```python
from build123d import *

# Parameters (mm, degrees)
SKETCH_W               = 7.5
SKETCH_H               = 7.5
PAD_DEPTH              = 10
POCKET_DEPTH           = 7.501
LINEARPATTERN_COUNT    = 2
LINEARPATTERN_PITCH    = 2.4
LINEARPATTERN001_COUNT = 2
LINEARPATTERN001_PITCH = 2.4
FILLET_R               = 0.175


with BuildPart() as part:
    # Sketch → Pad (new body)
    with BuildSketch(Plane.XY):
        Rectangle(SKETCH_W, SKETCH_H)
    extrude(amount=PAD_DEPTH)

    # Sketch001 (on Face2 of Pad) → Pocket (cut, through all)
    with BuildSketch(Plane.XZ.offset(3.75)):
        Polygon((-1, 10.1), (0, 10.1), (1, 10.1), (0.5, 2), (0, 2), (-0.5, 2), align=None)
    pocket = extrude(amount=-POCKET_DEPTH, mode=Mode.SUBTRACT)

    # LinearPattern: Pocket ×2
    with Locations(*[(i * LINEARPATTERN_PITCH, 0, 0) for i in range(1, LINEARPATTERN_COUNT)]):
        add(pocket, mode=Mode.SUBTRACT)

    # LinearPattern001: Pocket ×2
    with Locations(*[(-i * LINEARPATTERN001_PITCH, 0, 0) for i in range(1, LINEARPATTERN001_COUNT)]):
        add(pocket, mode=Mode.SUBTRACT)

    # Fillet
    fillet_edges = [part.edges().sort_by_distance(p)[0] for p in [
        (-3.75, 0, 10),
        (-3.393827, 0, 10),
        (-1.406173, 0, 10),
        (-0.993827, 0, 10),
        (0.993827, 0, 10),
        (1.406173, 0, 10),
        (3.393827, 0, 10),
        (3.75, 0, 10),
        (-2.9, 0, 2),
        (-0.5, 0, 2),
        (1.9, 0, 2),
        (3.75, 0, 0),
        (-3.75, 0, 0),
        (-1.9, 0, 2),
        (0.5, 0, 2),
        (2.9, 0, 2),
    ]]
    fillet(fillet_edges, radius=FILLET_R)


solid = part.part
```
Work out the finished part from the listing and answer in its coordinate system (mm). A direction names the side the tool comes from. Coordinates: 2 decimals unless noted, no trailing zeros. Loops run counter-clockwise (first coordinate to the right, second up) from the corner with the lowest first, then second, coordinate; pieces in that order, holes last. Notation, with made-up numbers: (-19.75, -22.75) -> (-12.75, -22.75) arc R24 ccw to (-12.75, 14.25) -> close; hole circle Ø1 at (64.25, -39). An arc over 180 degrees is marked (long way). Answer as CSV lines item,"result".
Q1. The part is cut by section A-A on z = 8. Write down the section's boundary in (x, y), and give its area (3 significant figures).
Findings:
outline,"(-3.75, -3.75) -> (-3.27, -3.75) -> (-3.27, 3.75) -> (-3.75, 3.75) -> close; (-1.53, -3.75) -> (-0.87, -3.75) -> (-0.87, 3.75) -> (-1.53, 3.75) -> close; (0.87, -3.75) -> (1.53, -3.75) -> (1.53, 3.75) -> (0.87, 3.75) -> close; (3.27, -3.75) -> (3.75, -3.75) -> (3.75, 3.75) -> (3.27, 3.75) -> close"
area,"17.1 mm²"
Q2. For a pull along X with two mould halves and no side action, classify faces 3 (the face through (-1, 3.75, 4)), 4 (the face through (-0.744, -0.052, 5.946)), 5 (the face through (3.75, 0, 5)) as +X half, -X half, draft (parallel to the pull), parting line (faces both ways), or undercut.
Findings:
face 3,"draft"
face 4,"undercut"
face 5,"+X half"
Q3. Find the intervals of material crossed by probe 1 along X at (y, z) = (1.5, 3); probe 2 along X at (y, z) = (-1.5, 5.75); probe 3 along Z at (x, y) = (-2.75, -2.5), in increasing order.
Findings:
probe 1,"x = -3.75 to -2.96, -1.84 to -0.56, 0.56 to 1.84, 2.96 to 3.75"
probe 2,"x = -3.75 to -3.13, -1.67 to -0.73, 0.73 to 1.67, 3.13 to 3.75"
probe 3,"z = 0 to 2"
Q4. A tool of negligible diameter and unlimited length cuts with its end or side. For faces 1 (the face through (3.15, -0.05, 6.05)), 2 (the face through (-3.75, 0, 5)), from which of +Z, -Z, +X, -X, +Y, -Y can it reach the whole face along a straight path? Write none if from no direction.
Findings:
face 1,"+Z, +Y, -Y"
face 2,"+Z, -Z, -X, +Y, -Y"
Q5. The part is cut by section C-C on x = -2.5. Write down the section's boundary in (y, z).
Findings:
outline,"(-3.75, 0) -> (3.75, 0) -> (3.75, 2) -> (-3.75, 2) -> close"
Q6. Each of these flat-tipped pins is pushed along its axis until it touches: pin 1 (0.5 mm diameter, centred on x = 0, y = 0.5, fed in from +Z); pin 2 (1.5 mm diameter, centred on x = 2.5, z = 9, fed in from -Y). Where does it stop, or does it pass through?
Findings:
pin 1,"stops at z = 2"
pin 2,"passes through"
Q7. The part is cut by section D-D on z = 4.5. Write down the section's boundary in (x, y).
Findings:
outline,"(-3.75, -3.75) -> (-3.05, -3.75) -> (-3.05, 3.75) -> (-3.75, 3.75) -> close; (-1.75, -3.75) -> (-0.65, -3.75) -> (-0.65, 3.75) -> (-1.75, 3.75) -> close; (0.65, -3.75) -> (1.75, -3.75) -> (1.75, 3.75) -> (0.65, 3.75) -> close; (3.05, -3.75) -> (3.75, -3.75) -> (3.75, 3.75) -> (3.05, 3.75) -> close"
